```python
from build123d import *

# Parameters (mm, degrees)
SKETCH1_R           = 1.25
BOSS_EXTRUDE1_DEPTH = 5
SKETCH2_R           = 1.25
CUT_EXTRUDE1_DEPTH  = 15
SKETCH3_R           = 1.5
CUT_EXTRUDE2_DEPTH  = 115
SKETCH4_R           = 1.5
CUT_EXTRUDE3_DEPTH  = 25
SKETCH5_R           = 1.5
CUT_EXTRUDE4_DEPTH  = 115
SKETCH6_R           = 1.5
CUT_EXTRUDE5_DEPTH  = 76
SKETCH8_R           = 1.5
CUT_EXTRUDE6_DEPTH  = 11


with BuildPart() as part:
    # Sketch1 → Boss-Extrude1 (new body)
    with BuildSketch(Plane.XY):
        with BuildLine():
            Line((-84, 0), (0, 0))
            Line((0, 0), (76, 0))
            Line((76, 0), (76, 5))
            Line((76, 5), (67, 5))
            ThreePointArc((67, 5), (64.87868, 5.87868), (64, 8))
            Line((64, 8), (64, 12))
            Line((64, 12), (47.5, 12))
            Line((47.5, 12), (47.5, 16.356013))
            ThreePointArc((47.5, 16.356013), (46.62132, 18.477334), (44.5, 19.356013))
            Line((44.5, 19.356013), (42.584405, 19.356013))
            Line((42.584405, 19.356013), (34.826345, 19.356013))
            Line((34.826345, 19.356013), (25.975089, 49.998488))
            ThreePointArc((25.975089, 49.998488), (25.952083, 51.579328), (26.735936, 52.952339))
            Line((26.735936, 52.952339), (57.374113, 83.590516))
            Line((57.374113, 83.590516), (60.374113, 83.590516))
            ThreePointArc((60.374113, 83.590516), (63.374113, 86.590516), (60.374113, 89.590516))
            Line((60.374113, 89.590516), (16.794783, 89.590516))
            ThreePointArc((16.794783, 89.590516), (14.991674, 90.192851), (13.912615, 91.757985))
            Line((13.912615, 91.757985), (11.538218, 99.977992))
            ThreePointArc((11.538218, 99.977992), (11.667419, 100.680829), (12.306797, 101))
            Line((12.306797, 101), (17.144141, 101))
            Line((17.144141, 101), (17.144141, 106))
            Line((17.144141, 106), (-17.144141, 106))
            Line((-17.144141, 106), (-17.144141, 101))
            Line((-17.144141, 101), (-12.306797, 101))
            ThreePointArc((-12.306797, 101), (-11.667419, 100.680829), (-11.538218, 99.977992))
            Line((-11.538218, 99.977992), (-28.574354, 41))
            Line((-28.574354, 41), (-64, 41))
            Line((-64, 41), (-64, 15))
            ThreePointArc((-64, 15), (-66.928932, 7.928932), (-74, 5))
            Line((-74, 5), (-84, 5))
            Line((-84, 5), (-84, 0))
        make_face()
        with Locations((0, 102.5)):
            Circle(SKETCH1_R, mode=Mode.SUBTRACT)
        with Locations((45, 17)):
            Circle(SKETCH1_R, mode=Mode.SUBTRACT)
        with Locations((41.5, 9)):
            Circle(SKETCH1_R, mode=Mode.SUBTRACT)
        with Locations((60.5, 9)):
            Circle(SKETCH1_R, mode=Mode.SUBTRACT)
        with Locations((60.374113, 86.590516)):
            Circle(SKETCH1_R, mode=Mode.SUBTRACT)
        with BuildLine():
            Line((-55, 35), (-34.296706, 35))
            ThreePointArc((-34.296706, 35), (-31.899041, 33.803109), (-31.414538, 31.167469))
            Line((-31.414538, 31.167469), (-36.325087, 14.167469))
            ThreePointArc((-36.325087, 14.167469), (-37.404145, 12.602335), (-39.207254, 12))
            Line((-39.207254, 12), (-55, 12))
            ThreePointArc((-55, 12), (-57.12132, 12.87868), (-58, 15))
            Line((-58, 15), (-58, 32))
            ThreePointArc((-58, 32), (-57.12132, 34.12132), (-55, 35))
        make_face(mode=Mode.SUBTRACT)
        with BuildLine():
            Line((-26.196215, 12), (25.838936, 12))
            ThreePointArc((25.838936, 12), (28.233641, 13.192962), (28.723818, 15.823077))
            Line((28.723818, 15.823077), (28.41252, 16.914174))
            Line((28.41252, 16.914174), (1.505858, 47.697877))
            ThreePointArc((1.505858, 47.697877), (0, 48.381673), (-1.505858, 47.697877))
            Line((-1.505858, 47.697877), (-28.940396, 16.310236))
            Line((-28.940396, 16.310236), (-29.078383, 15.832531))
            ThreePointArc((-29.078383, 15.832531), (-28.59388, 13.196891), (-26.196215, 12))
        make_face(mode=Mode.SUBTRACT)
        with BuildLine():
            Line((15.437427, 62.39185), (24.030004, 32.274885))
            ThreePointArc((24.030004, 32.274885), (23.062279, 29.969192), (20.600891, 30.409964))
            Line((20.600891, 30.409964), (3.142654, 50.383797))
            ThreePointArc((3.142654, 50.383797), (2.648512, 51.7), (3.142654, 53.016203))
            Line((3.142654, 53.016203), (12.008314, 63.159336))
            ThreePointArc((12.008314, 63.159336), (13.950994, 63.794846), (15.437427, 62.39185))
        make_face(mode=Mode.SUBTRACT)
        with BuildLine():
            Line((-3.142654, 53.016203), (-12.152635, 63.324452))
            ThreePointArc((-12.152635, 63.324452), (-14.092115, 63.960676), (-15.579938, 62.563269))
            Line((-15.579938, 62.563269), (-24.47463, 31.770424))
            ThreePointArc((-24.47463, 31.770424), (-23.511594, 29.459997), (-21.047327, 29.8992))
            Line((-21.047327, 29.8992), (-3.142654, 50.383797))
            ThreePointArc((-3.142654, 50.383797), (-2.648512, 51.7), (-3.142654, 53.016203))
        make_face(mode=Mode.SUBTRACT)
        with BuildLine():
            Line((-13.270648, 70.557882), (-5.969919, 95.832531))
            ThreePointArc((-5.969919, 95.832531), (-4.89086, 97.397665), (-3.087751, 98))
            Line((-3.087751, 98), (3.014386, 98))
            ThreePointArc((3.014386, 98), (4.821424, 97.394706), (5.899268, 95.823077))
            Line((5.899268, 95.823077), (13.149527, 70.410935))
            ThreePointArc((13.149527, 70.410935), (13.177986, 69.425395), (12.73213, 68.546014))
            Line((12.73213, 68.546014), (1.505858, 55.702123))
            ThreePointArc((1.505858, 55.702123), (0, 55.018327), (-1.505858, 55.702123))
            Line((-1.505858, 55.702123), (-12.855061, 68.686658))
            ThreePointArc((-12.855061, 68.686658), (-13.30163, 69.569239), (-13.270648, 70.557882))
        make_face(mode=Mode.SUBTRACT)
        with BuildLine():
            Line((17.892665, 77.979312), (17.361692, 79.621616))
            ThreePointArc((17.361692, 79.621616), (17.795471, 82.341157), (20.249686, 83.590516))
            Line((20.249686, 83.590516), (45.888831, 83.590516))
            ThreePointArc((45.888831, 83.590516), (48.66047, 81.738566), (48.010152, 78.469195))
            Line((48.010152, 78.469195), (28.190525, 58.649569))
            ThreePointArc((28.190525, 58.649569), (25.327066, 57.864134), (23.190599, 59.926126))
            Line((23.190599, 59.926126), (17.892665, 77.979312))
        make_face(mode=Mode.SUBTRACT)
    extrude(amount=BOSS_EXTRUDE1_DEPTH)

    # Sketch2 → Cut-Extrude1 (cut)
    with BuildSketch(Plane.XY.offset(5)):
        with Locations((-33.5, 5)):
            Circle(SKETCH2_R)
        with Locations((-60.5, 5)):
            Circle(SKETCH2_R)
    extrude(amount=-CUT_EXTRUDE1_DEPTH, mode=Mode.SUBTRACT)

    # Sketch3 → Cut-Extrude2 (cut)
    with BuildSketch(Plane(origin=(0, 106, 0), x_dir=(1, 0, 0), z_dir=(0, 1, 0))):
        with Locations(Location((-80, -2.5, 0), (0, 0, 270))):
            Circle(SKETCH3_R)
    extrude(amount=-CUT_EXTRUDE2_DEPTH, mode=Mode.SUBTRACT)

    # Sketch4 → Cut-Extrude3 (cut)
    with BuildSketch(Plane(origin=(0, 106, 0), x_dir=(1, 0, 0), z_dir=(0, 1, 0))):
        with Locations(Location((45.5, -2.5, 0), (0, 0, 285.023837))):
            Circle(SKETCH4_R)
        with Locations(Location((56.5, -2.5, 0), (0, 0, 305.643618))):
            Circle(SKETCH4_R)
    extrude(amount=-CUT_EXTRUDE3_DEPTH, mode=Mode.SUBTRACT)

    # Sketch5 → Cut-Extrude4 (cut)
    with BuildSketch(Plane(origin=(0, 106, 0), x_dir=(1, 0, 0), z_dir=(0, 1, 0))):
        with Locations(Location((72, -2.5, 0), (0, 0, 270))):
            Circle(SKETCH5_R)
    extrude(amount=-CUT_EXTRUDE4_DEPTH, mode=Mode.SUBTRACT)

    # Sketch6 → Cut-Extrude5 (cut)
    with BuildSketch(Plane(origin=(0, 106, 0), x_dir=(1, 0, 0), z_dir=(0, 1, 0))):
        with Locations(Location((-42, -2.5, 0), (0, 0, 180))):
            Circle(SKETCH6_R)
        with Locations(Location((-60, -2.5, 0), (0, 0, 270))):
            Circle(SKETCH6_R)
    extrude(amount=-CUT_EXTRUDE5_DEPTH, mode=Mode.SUBTRACT)

    # Sketch8 → Cut-Extrude6 (cut)
    with BuildSketch(Plane(origin=(0, 106, 0), x_dir=(1, 0, 0), z_dir=(0, 1, 0))):
        with Locations(Location((-9, -2.5, 0), (0, 0, 270))):
            Circle(SKETCH8_R)
        with Locations(Location((9, -2.5, 0), (0, 0, 270))):
            Circle(SKETCH8_R)
    extrude(amount=-CUT_EXTRUDE6_DEPTH, mode=Mode.SUBTRACT)


solid = part.part
```
Can you work these out from the model? Positions are in its coordinate system, mm. A direction names the side the tool comes from. Coordinates: 2 decimals unless noted, no trailing zeros. Write each loop counter-clockwise with the first axis right and the second up, starting at its lowest first coordinate (ties: lowest second). Pieces come first, ordered by that corner, then holes. Notation, with made-up numbers: (-39, 46) - (-8, 46) arc R16 cw to (-8, 56) - close; hole circle Ø9 at (44, 73.5). An arc over 180 degrees is marked (long way). Return JSON: item names as keys, results as strings.
Q1. Thinking about a two-plate mould opening in Y: for faces 1 (the flat face through (-46, 41, 2)), 2 (the flat face through (-19.937, 70.902, 2.465)), 3 (the cylindrical face through (-10.464, 100.577, 2.175)), which applies, +Y half, -Y half, draft (parallel to the pull), parting line (faces both ways), or undercut?
Computed values:
{"face 1": "+Y half", "face 2": "undercut", "face 3": "draft"}
Q2. On a 3-axis mill with a long thin cutter (end or side, diameter ignored), from which of +Z, -Z, +X, -X, +Y, -Y can I reach the whole of each face in a straight line? I mean faces 4 (the cylindrical face through (15.01, 90.18, 2.46)), 5 (the flat face through (-9, 95, 2)), 6 (the flat face through (-78, 5, 2)), 7 (the cylindrical face through (-14.063, 63.967, 2.465)). Say none if no direction works.
Computed values:
{"face 4": "+Z, -Z, +X", "face 5": "+Y", "face 6": "+Z, -Z, -X, +Y", "face 7": "+Z, -Z"}
Q3. If we section it at A-A (x = 37.5): Please give me the cut outline in (y, z), then the cut area to 3 significant figures.
Computed values:
{"outline": "(0, 0) - (19.36, 0) - (19.36, 5) - (0, 5) - close; (63.72, 0) - (67.96, 0) - (67.96, 5) - (63.72, 5) - close; (83.59, 0) - (89.59, 0) - (89.59, 5) - (83.59, 5) - close", "area": "148 mm2"}
Q4. Please list where these lines run through material, in increasing order: L1, parallel to X at y = 2.75, z = 2.5; L2, parallel to Y at x = 55, z = 1.7; L3, parallel to X at y = 10, z = 1.75. Write a range as from..to.
Computed values:
{"L1": "x = -84..-81.5, -78.5..70.5, 73.5..76", "L2": "y = 0..12, 81.22..89.59", "L3": "x = -65.34..40.75, 42.25..59.75, 61.25..64"}
Q5. I'm going to push flat-ended pins straight in: pin 1 Ø2.5 at (x, z) = (71, 1.5) entering from +Y; pin 2 Ø1.5 at (x, z) = (8.5, 2) entering from +Y; pin 3 Ø1.5 at (y, z) = (23.5, 1.5) entering from -X. Where does each tip first touch, or does it pass through?
Computed values:
{"pin 1": "stops at y = 5", "pin 2": "stops at y = 95", "pin 3": "stops at x = -64"}
